from build123d import *

# Parameters (mm, degrees)
SKETCH1_W                 = 127
SKETCH1_H                 = 76.2
BOSS_EXTRUDE1_DEPTH       = 12.7
BOSS_EXTRUDE2_DEPTH       = 12.7
BOSS_EXTRUDE2_DEPTH_BACK  = 12.7
SKETCH3_R                 = 3.81
CUT_EXTRUDE1_DEPTH        = 29.464
SKETCH4_W                 = 17.78
SKETCH4_H                 = 6.604
CUT_EXTRUDE2_DEPTH        = 29.464
BOSS_EXTRUDE3_START       = -12.7
BOSS_EXTRUDE3_OUTLINE_W   = 57.78
BOSS_EXTRUDE3_OUTLINE_H   = 32.76
BOSS_EXTRUDE3_OUTLINE_W_2 = 40
BOSS_EXTRUDE3_OUTLINE_H_2 = 20.06
BOSS_EXTRUDE3_DEPTH       = 45.5
CUT_EXTRUDE5_DEPTH        = 44.196
SKETCH10_W                = 20.976278311
SKETCH10_H                = 20.06
BOSS_EXTRUDE5_DEPTH       = 12.7
CUT_EXTRUDE7_DEPTH        = 187.177258339
CUT_EXTRUDE7_DEPTH_BACK   = 76.2
SKETCH11_W                = 20.06
SKETCH11_H                = 7.443830751
SPLIT1_START              = 12.7
SPLIT1_OUTLINE_W          = 57.78
SPLIT1_OUTLINE_H          = 32.76
SPLIT1_OUTLINE_W_2        = 40
SPLIT1_OUTLINE_H_2        = 20.06
SPLIT1_DEPTH              = 45.5
CUT_EXTRUDE9_DEPTH        = 24.384
SKETCH13_R                = 1.905
CUT_EXTRUDE10_DEPTH       = 36.83
SKETCH14_W                = 17.78
SKETCH14_H                = 0.127
CUT_EXTRUDE11_DEPTH       = 98.260775753
SKETCH15_W                = 17.78
SKETCH15_H                = 0.0635
CUT_EXTRUDE12_DEPTH       = 98.260775753
SKETCH16_W                = 17.78
SKETCH16_H                = 0.0635
CUT_EXTRUDE13_DEPTH       = 98.260775753
SKETCH17_W                = 17.78
SKETCH17_H                = 0.127
CUT_EXTRUDE14_DEPTH       = 98.260775753
SKETCH18_W                = 17.78
SKETCH18_H                = 0.0635
CUT_EXTRUDE15_DEPTH       = 98.260775753
SKETCH19_R                = 1.671154259
SKETCH19_R_2              = 1.733603543
SKETCH19_R_3              = 1.269040072
SKETCH19_R_4              = 1.545344409
CUT_EXTRUDE16_DEPTH       = 94.290987775


# Read off the part's stored shape, not the designer's step: Boss-Extrude3, Split1
with BuildPart() as part:
    # Sketch1 → Boss-Extrude1 (new body)
    with BuildSketch(Plane(origin=(0, 0, 0), x_dir=(1, 0, 0), z_dir=(0, 1, 0))):
        Rectangle(SKETCH1_W, SKETCH1_H)
    extrude(amount=BOSS_EXTRUDE1_DEPTH)

    # Sketch2 → Boss-Extrude2 (add, two sides: drawn at the far end of the back side and taken through both)
    with BuildSketch(Plane(origin=(0, 12.7, 0), x_dir=(1, 0, 0), z_dir=(0, 1, 0)).offset(-BOSS_EXTRUDE2_DEPTH_BACK)):
        with BuildLine():
            Line((72.39, 8.89), (63.5, 8.89))
            Line((63.5, 8.89), (48.26, 8.89))
            Line((48.26, 8.89), (48.26, -8.89))
            Line((48.26, -8.89), (63.5, -8.89))
            Line((63.5, -8.89), (72.39, -8.89))
            ThreePointArc((72.39, -8.89), (81.28, 0), (72.39, 8.89))
        make_face()
        with BuildLine():
            Line((-48.26, -8.89), (-63.5, -8.89))
            Line((-63.5, -8.89), (-72.39, -8.89))
            ThreePointArc((-72.39, -8.89), (-81.28, 0), (-72.39, 8.89))
            Line((-72.39, 8.89), (-63.5, 8.89))
            Line((-63.5, 8.89), (-48.26, 8.89))
            Line((-48.26, 8.89), (-48.26, -8.89))
        make_face()
    extrude(amount=BOSS_EXTRUDE2_DEPTH + BOSS_EXTRUDE2_DEPTH_BACK)

    # Sketch3 → Cut-Extrude1 (cut)
    with BuildSketch(Plane(origin=(0, 25.4, 0), x_dir=(1, 0, 0), z_dir=(0, 1, 0))):
        with Locations(Location((72.613721689, 0, 0), (0, 0, 270))):
            Circle(SKETCH3_R)
        with Locations(Location((-72.613721689, 0, 0), (0, 0, 90))):
            Circle(SKETCH3_R)
    extrude(amount=-CUT_EXTRUDE1_DEPTH, mode=Mode.SUBTRACT)

    # Sketch4 → Cut-Extrude2 (cut)
    with BuildSketch(Plane.XY.offset(8.89)):
        with Locations((72.39, 22.098)):
            Rectangle(SKETCH4_W, SKETCH4_H)
        with Locations((72.39, 9.398)):
            Rectangle(SKETCH4_W, SKETCH4_H)
        with Locations((-72.39, 9.398)):
            Rectangle(SKETCH4_W, SKETCH4_H)
        with Locations((-72.39, 22.098)):
            Rectangle(SKETCH4_W, SKETCH4_H)
    extrude(amount=-CUT_EXTRUDE2_DEPTH, mode=Mode.SUBTRACT)



with BuildPart() as body_2:
    # Boss-Extrude3 outline → Boss-Extrude3 (new body)
    with BuildSketch(Plane(origin=(0, 25.4, 0), x_dir=(1, 0, 0), z_dir=(0, 1, 0)).offset(BOSS_EXTRUDE3_START)):
        with Locations((62.523721689, 0)):
            Rectangle(BOSS_EXTRUDE3_OUTLINE_W, BOSS_EXTRUDE3_OUTLINE_H)
        with Locations((62.523721689, 0)):
            Rectangle(BOSS_EXTRUDE3_OUTLINE_W_2, BOSS_EXTRUDE3_OUTLINE_H_2, mode=Mode.SUBTRACT)
    extrude(amount=BOSS_EXTRUDE3_DEPTH)

    # Sketch7 → Cut-Extrude5 (cut)
    with BuildSketch(Plane.XY.offset(16.38)):
        with BuildLine():
            Line((91.413721689, 45.5), (91.413721689, 12.7))
            Line((91.413721689, 12.7), (63.5, 12.7))
            add(Edge.make_bspline(
                [(91.413721689, 45.5), (71.582716482, 29.1), (63.5, 12.7)],
                knots=[0, 0, 0, 1, 1, 1], degree=2, weights=[1, 3, 1]))
        make_face()
    extrude(amount=-CUT_EXTRUDE5_DEPTH, mode=Mode.SUBTRACT)


with BuildPart() as part_1:
    add(part.part)

    add(body_2.part)  # Boss-Extrude5 merges body 2
    # Sketch10 → Boss-Extrude5 (add)
    with BuildSketch(Plane(origin=(0, 12.7, 0), x_dir=(1, 0, 0), z_dir=(0, 1, 0))):
        with Locations((53.011860845, 0)):
            Rectangle(SKETCH10_W, SKETCH10_H)
        with Locations((-53.011860845, 0)):
            Rectangle(SKETCH10_W, SKETCH10_H)
    extrude(amount=BOSS_EXTRUDE5_DEPTH)

    # Sketch11 → Cut-Extrude7 (cut, two sides: drawn at the far end of the back side and taken through both)
    with BuildSketch(Plane(origin=(91.413721689, 0, 0), x_dir=(0, 0, -1), z_dir=(1, 0, 0)).offset(-CUT_EXTRUDE7_DEPTH_BACK)):
        with Locations((0, 41.778084624)):
            Rectangle(SKETCH11_W, SKETCH11_H)
    extrude(amount=CUT_EXTRUDE7_DEPTH + CUT_EXTRUDE7_DEPTH_BACK, mode=Mode.SUBTRACT)

    # Split1 outline → Split1 (cut)
    with BuildSketch(Plane(origin=(0, 0, 0), x_dir=(1, 0, 0), z_dir=(0, 1, 0)).offset(SPLIT1_START)):
        with Locations((62.523721689, 0)):
            Rectangle(SPLIT1_OUTLINE_W, SPLIT1_OUTLINE_H)
        with Locations((62.523721689, 0)):
            Rectangle(SPLIT1_OUTLINE_W_2, SPLIT1_OUTLINE_H_2, mode=Mode.SUBTRACT)
    extrude(amount=SPLIT1_DEPTH, mode=Mode.SUBTRACT)

    # Sketch12 → Cut-Extrude9 (cut)
    with BuildSketch(Plane(origin=(0, 12.7, 0), x_dir=(1, 0, 0), z_dir=(0, 1, 0))):
        with BuildLine():
            Line((63.5, 38.1), (44.45, 38.1))
            ThreePointArc((44.45, 38.1), (57.920384182, 32.520384182), (63.5, 19.05))
            Line((63.5, 19.05), (63.5, 38.1))
        make_face()
        with BuildLine():
            Line((63.5, -38.1), (63.5, -19.05))
            ThreePointArc((63.5, -19.05), (57.920384182, -32.520384182), (44.45, -38.1))
            Line((44.45, -38.1), (63.5, -38.1))
        make_face()
        with BuildLine():
            Line((-63.5, -38.1), (-44.45, -38.1))
            ThreePointArc((-44.45, -38.1), (-57.920384182, -32.520384182), (-63.5, -19.05))
            Line((-63.5, -19.05), (-63.5, -38.1))
        make_face()
        with BuildLine():
            ThreePointArc((-63.5, 19.05), (-57.920384182, 32.520384182), (-44.45, 38.1))
            Line((-44.45, 38.1), (-63.5, 38.1))
            Line((-63.5, 38.1), (-63.5, 19.05))
        make_face()
    extrude(amount=-CUT_EXTRUDE9_DEPTH, mode=Mode.SUBTRACT)

    # Sketch13 → Cut-Extrude10 (cut)
    with BuildSketch(Plane(origin=(0, 0, -10.03), x_dir=(-1, 0, 0), z_dir=(0, 0, -1))):
        with Locations((56.9735, 16.002)):
            Circle(SKETCH13_R)
        with Locations((49.3535, 16.002)):
            Circle(SKETCH13_R)
    cut_extrude10 = extrude(amount=-CUT_EXTRUDE10_DEPTH, mode=Mode.SUBTRACT)

    # Mirror1: Cut-Extrude10 across plane
    add(cut_extrude10.mirror(Plane(origin=(0, 0, 0), x_dir=(0, 0, 1), z_dir=(1, 0, 0))), mode=Mode.SUBTRACT)

    # Sketch14 → Cut-Extrude11 (cut, through all)
    with BuildSketch(Plane(origin=(0, 0, -8.89), x_dir=(-1, 0, 0), z_dir=(0, 0, -1))):
        with Locations((72.39, 6.0325)):
            Rectangle(SKETCH14_W, SKETCH14_H)
    extrude(amount=-CUT_EXTRUDE11_DEPTH, mode=Mode.SUBTRACT)

    # Sketch15 → Cut-Extrude12 (cut, through all)
    with BuildSketch(Plane(origin=(0, 0, -8.89), x_dir=(-1, 0, 0), z_dir=(0, 0, -1))):
        with Locations((72.39, 18.76425)):
            Rectangle(SKETCH15_W, SKETCH15_H)
    extrude(amount=-CUT_EXTRUDE12_DEPTH, mode=Mode.SUBTRACT)

    # Sketch16 → Cut-Extrude13 (cut, through all)
    with BuildSketch(Plane(origin=(0, 0, -8.89), x_dir=(-1, 0, 0), z_dir=(0, 0, -1))):
        with Locations((72.39, 12.73175)):
            Rectangle(SKETCH16_W, SKETCH16_H)
    extrude(amount=-CUT_EXTRUDE13_DEPTH, mode=Mode.SUBTRACT)

    # Sketch17 → Cut-Extrude14 (cut, through all)
    with BuildSketch(Plane(origin=(0, 0, -8.89), x_dir=(-1, 0, 0), z_dir=(0, 0, -1))):
        with Locations((-72.39, 6.0325)):
            Rectangle(SKETCH17_W, SKETCH17_H)
    extrude(amount=-CUT_EXTRUDE14_DEPTH, mode=Mode.SUBTRACT)

    # Sketch18 → Cut-Extrude15 (cut, through all)
    with BuildSketch(Plane(origin=(0, 0, -8.89), x_dir=(-1, 0, 0), z_dir=(0, 0, -1))):
        with Locations((-72.39, 12.73175)):
            Rectangle(SKETCH18_W, SKETCH18_H)
        with Locations((-72.39, 18.76425)):
            Rectangle(SKETCH18_W, SKETCH18_H)
    extrude(amount=-CUT_EXTRUDE15_DEPTH, mode=Mode.SUBTRACT)

    # Sketch19 → Cut-Extrude16 (cut, through all)
    with BuildSketch(Plane(origin=(0, 0, 0), x_dir=(-1, 0, 0), z_dir=(0, -1, 0))):
        with Locations(Location((-32.09925, 24.511, 0), (0, 0, 90))):
            Circle(SKETCH19_R)
        with Locations(Location((25.90074068, 24.511, 0), (0, 0, 90))):
            Circle(SKETCH19_R_2)
        with Locations(Location((25.90074068, -24.511, 0), (0, 0, 90))):
            Circle(SKETCH19_R_3)
        with Locations(Location((-32.09925, -24.511, 0), (0, 0, 90))):
            Circle(SKETCH19_R_4)
    extrude(amount=-CUT_EXTRUDE16_DEPTH, mode=Mode.SUBTRACT)


solid = part_1.part
Can you work these out from the model? Positions are in its coordinate system, mm. A direction names the side the tool comes from. Give positions to 0.01 mm unless a question says otherwise; leave off trailing zeros. Order: outer loops, then holes, each group sorted by start corner. A loop starts at its lowest first (then second) coordinate and runs counter-clockwise, first axis right, second up. Notation, with made-up numbers: M -32,22.25 L 22,22.25 A25 cw 22,49.25 Z; hole C -16.75,-20.75 d8. An arc over 180 degrees is marked long. Use a Markdown table: item, result. Add a question column.
Item 1: Suppose I cut it at A-A (z = 0). Count the separate pieces of the cut face and the enclosed holes in it, then the cut area to 3 significant figures.
Item 2: We'd pull the mould along Y, two halves only. Please class faces 1 (the cylindrical face through (76.39, 3.03, -0.5)), 2 (the flat face through (-63.5, 12.5, 0.3)), 3 (the flat face through (-68, 18.732, 0)): +Y half, -Y half, draft (parallel to the pull), parting line (faces both ways), or undercut.
Item 3: Suppose I cut it at B-B (x = -32). List the corners of the cut face in (y, z) for me, then the cut area to 3 significant figures.
Item 4: Will these pins go through, and if not, where does the flat tip stop? pin 1 (5 mm diameter, centred on x = -56.97, y = 16, fed in from -Z); pin 2 (1.8 mm diameter, centred on x = -68.5, y = 15, fed in from -Z); pin 3 (5.5 mm diameter, centred on x = 75.5, z = -2.5, fed in from +Y).
Item 5: Suppose I cut it at C-C (z = 13). List the corners of the cut face in (x, y) for me.
Item 6: For faces 4 (the flat face through (68.6, 12.764, -0.1)), 5 (the flat face through (68.6, 18.732, -0.1)), 6 (the flat face through (-68, 16, -8.89)), which set-ups out of +Z, -Z, +X, -X, +Y, -Y let a thin tool reach every point of the face, with its end or its side?
Item 7: If I drill on L1, parallel to X at y = 5.25, z = -24.5; L2, parallel to Z at x = -27, y = 4.25; L3, parallel to X at y = 16.5, z = 4, over which ranges is the centre line in solid material (lowest first)? Write a range as [from, to].
Answer sheet:
| question | item | result |
|---|---|---|
| 1 | separate pieces | 5 |
| 1 | enclosed holes | 4 |
| 1 | area | 2,340 mm² |
| 2 | face 1 | draft |
| 2 | face 2 | undercut |
| 2 | face 3 | +Y half |
| 3 | outline | M 0,-38.1 L 12.7,-38.1 L 12.7,38.1 L 0,38.1 Z |
| 3 | area | 968 mm² |
| 4 | pin 1 | stops at z = -10.03 |
| 4 | pin 2 | stops at z = -8.89 |
| 4 | pin 3 | stops at y = 18.73 |
| 5 | outline | M -63.5,0 L 63.5,0 L 63.5,12.7 L -63.5,12.7 Z |
| 6 | face 4 | +Z, -Z, +X |
| 6 | face 5 | +Z, -Z, +X, +Y |
| 6 | face 6 | -Z, -X, +Y, -Y |
| 7 | L1 | x = [-62.7, -27.63], [-24.17, 30.43], [33.77, 62.7] |
| 7 | L2 | z = [-38.1, -25.85], [-23.17, 23.88], [25.15, 38.1] |
| 7 | L3 | x = [-80.33, -58.81], [-55.13, -51.19], [-47.51, -42.52], [42.52, 47.51], [51.19, 55.13], [58.81, 80.33] |
